Check sheet for the modelled part. Datum: model origin and axes. Units: mm. Face numbers are marked on the shaded views. Coordinates: 2 decimals unless noted, no trailing zeros. Order: outer loops, then holes, each group sorted by start corner. A loop starts at its lowest first (then second) coordinate and runs counter-clockwise, first axis right, second up.
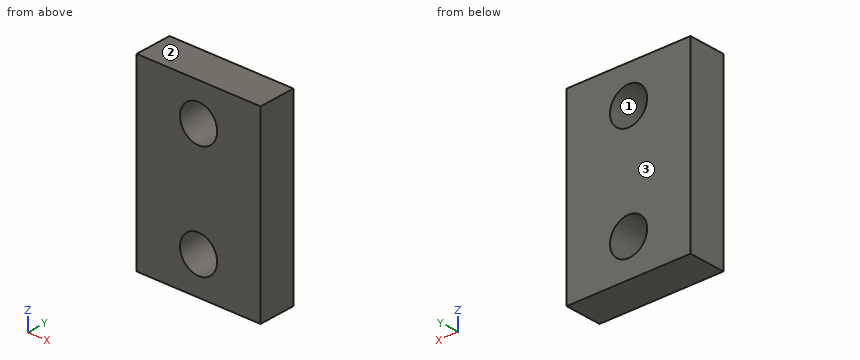
Autodesk Inventor part; units mm, degrees
ref_plane "YZ Plane" through (0, 0, 0) normal (1, 0, 0) x (0, 1, 0)
ref_plane "XZ Plane" through (0, 0, 0) normal (0, 1, 0) x (-1, 0, 0)
ref_plane "XY Plane" through (0, 0, 0) normal (0, 0, 1) x (1, 0, 0)
sketch "Sketch1" plane through (0, 0, 0) normal (0, 1, 0) x (-1, 0, 0)
  line L0 (5, -7.5) -> (-5, -7.5)
  line L1 (-5, -7.5) -> (-5, 7.5)
  line L2 (-5, 7.5) -> (5, 7.5)
  line L3 (5, 7.5) -> (5, -7.5)
  line L4 (5, -7.5) -> (-5, 7.5) construction
  line L5 (-5, -7.5) -> (5, 7.5) construction
  circle A0 centre (0, -4.5) radius 1.5
  circle A1 centre (0, 4.5) radius 1.5
  line L6 (0, 4.5) -> (0, 7.5) construction
  line L7 (0, -7.5) -> (0, -4.5) construction
  point P0 (0, 0)
  dimension "d0" = 10
  dimension "d1" = 15
  dimension "d2" = 3
  dimension "d3" = 3
  dimension "d4" = 9
  dimension "d5" = 5
  dimension "d7" = 5
extrude "Extrusion1" add sketch "Sketch1" along normal blind 3
equation "\"d5\" = 0.5 * d0"
equation "\"d7\" = d5"
properties part number "thumper-bumper-plunger-interface"
(1) Cross-section at B-B (x = 0). Enter the section's corners in (y, z), and give its area (3 significant figures).
Filled in:
outline: (0, -7.5) - (3, -7.5) - (3, -6) - (0, -6) - close; (0, -3) - (3, -3) - (3, 3) - (0, 3) - close; (0, 6) - (3, 6) - (3, 7.5) - (0, 7.5) - close
area: 27.0 mm2
(2) Cross-section at C-C (y = 2.7). Enter the section's corners in (x, z).
Filled in:
outline: (-5, -7.5) - (5, -7.5) - (5, 7.5) - (-5, 7.5) - close; hole circle Ø3 at (0, -4.5); hole circle Ø3 at (0, 4.5)
(3) Release check for a two-part mould opening along Z. For the marked faces 1, 2 and 3 record: +Z half, -Z half, draft (parallel to the pull), parting line (faces both ways), or undercut.
Filled in:
face 1: undercut
face 2: +Z half
face 3: draft
(4) Thickness scan on probe 1 along Z at (x, y) = (0, 2.2); probe 2 along Z at (x, y) = (-1, 0.9); probe 3 along X at (y, z) = (0.85, 3.75). Record the ranges inside material, lowest first.
Filled in:
probe 1: z = -7.5 to -6, -3 to 3, 6 to 7.5
probe 2: z = -7.5 to -5.62, -3.38 to 3.38, 5.62 to 7.5
probe 3: x = -5 to -1.3, 1.3 to 5
(5) Cross-section at A-A (z = 4.5). Enter the section's corners in (x, y), and give its area (3 significant figures).
Filled in:
outline: (-5, 0) - (-1.5, 0) - (-1.5, 3) - (-5, 3) - close; (1.5, 0) - (5, 0) - (5, 3) - (1.5, 3) - close
area: 21.0 mm2
